Geometry check sheet. Reference: the model listing, model coordinates, mm. Face numbers are marked on the shaded views. A direction names the side the tool comes from. Give positions to 0.01 mm unless a question says otherwise; leave off trailing zeros. Write each loop counter-clockwise with the first axis right and the second up, starting at its lowest first coordinate (ties: lowest second). Pieces come first, ordered by that corner, then holes. Notation, with made-up numbers: M -37,31.25 L -23,31.25 A32 ccw -23,69.25 Z; hole C 8,82.25 d7. An arc over 180 degrees is marked long. One line per item, written item: value. Start each with the question number.
1. Tool access check on the marked faces 1, 2 and 3. Record the directions out of +Z, -Z, +X, -X, +Y, -Y that give a thin tool (end or side, any length) a straight path to the whole face; none if there is none.
2. Cross-section at C-C on z = -3. Record the cut outline in (x, y).
3. Cross-section at A-A on x = 94. Record the cut outline in (y, z) (3 decimals), then the cut area to 4 significant figures.
4. Cross-section at B-B on y = 4.5. Record the cut outline in (x, z) (3 decimals).
5. Scan lines: line 1 (Y direction, x = 6, z = 2.2) (3 decimals); line 2 (Y direction, x = 94, z = 4.2); line 3 (Z direction, x = 62.5, y = 10.75). Record each from-to range of solid material in increasing order.
6. Gauge pin test, flat ends, axial feed: pin 1 (3.5 mm diameter, centred on y = 5.5, z = -1.5, fed in from +X); pin 2 (6 mm diameter, centred on y = 2, z = -4, fed in from +X); pin 3 (5 mm diameter, centred on y = 8, z = -4.5, fed in from -X); pin 4 (4.5 mm diameter, centred on x = 91.5, y = 3, fed in from -Z). Record the tip position at first contact, or that the pin passes through.
Autodesk Inventor part; units mm, degrees
ref_plane "YZ Plane" through (0, 0, 0) normal (1, 0, 0) x (0, 1, 0)
ref_plane "XZ Plane" through (0, 0, 0) normal (0, 1, 0) x (-1, 0, 0)
ref_plane "XY Plane" through (0, 0, 0) normal (0, 0, 1) x (1, 0, 0)
sketch "Sketch1" plane through (0, 0, 0) normal (0, 0, 1) x (1, 0, 0)
  line L0 (0, 0) -> (100, 0)
  line L1 (100, 0) -> (100, 9)
  line L2 (88, 12) -> (12, 12)
  line L3 (0, 9) -> (0, 0)
  line L4 (12, 12) -> (12, 9)
  line L5 (12, 9) -> (0, 9)
  line L6 (88, 12) -> (88, 9)
  line L7 (88, 9) -> (100, 9)
  dimension "d6" = 100
  dimension "d7" = 3
  dimension "d8" = 3
  dimension "d9" = 12
  dimension "d10" = 12
  dimension "d11" = 9
  dimension "d12" = 9
  dimension "d13" = 12
extrude "Extrusion1" add sketch "Sketch1" along normal blind 6
sketch "Sketch2" plane through (0, 0, 0) normal (0, 0, -1) x (-1, 0, 0)
  line L0 (-88, 12) -> (-12, 12)
  line L1 (0, 0) -> (-100, 0)
  line L2 (-88, 12) -> (-12, 12)
  line L3 (-12, 12) -> (-12, 0)
  line L4 (-12, 0) -> (-88, 0)
  line L5 (-88, 0) -> (-88, 12)
extrude "Extrusion2" add sketch "Sketch2" along normal blind 6
sketch "Sketch3" plane through (0, 0, 0) normal (0, 0, -1) x (-1, 0, 0)
  circle A0 centre (-6, 4.5) radius 1.725
  line L0 (-12, 9) -> (0, 9)
  line L1 (0, 9) -> (0, 0)
  circle A1 centre (-94, 4.5) radius 1.725
  line L2 (-88, 0) -> (-100, 0)
  line L3 (-100, 0) -> (-100, 9)
  dimension "d18" = 3.45
  dimension "d19" = 4.5
  dimension "d20" = 6
  dimension "d21" = 3.45
  dimension "d22" = 4.5
  dimension "d23" = 6
extrude "Extrusion3" cut sketch "Sketch3" against normal blind 3
sketch "Sketch4" plane through (0, 0, 6) normal (0, 0, 1) x (1, 0, 0)
  circle A0 centre (6, 4.5) radius 3
  line L0 (12, 9) -> (0, 9)
  line L1 (0, 9) -> (0, 0)
  circle A1 centre (94, 4.5) radius 1.725
  circle A2 centre (94, 4.5) radius 3
  dimension "d26" = 6
  dimension "d27" = 4.5
  dimension "d28" = 6
  dimension "d29" = 6
extrude "Extrusion4" cut sketch "Sketch4" against normal blind 3 contours A0 | A1 | A2
fillet "Fillet1" radius 1.5 2 edges at (50, 12, 6) (50, 12, -6)
equation "\"d8\" = d7"
equation "\"d10\" = d9"
equation "\"d12\" = d11"
properties part number "beam10cm"
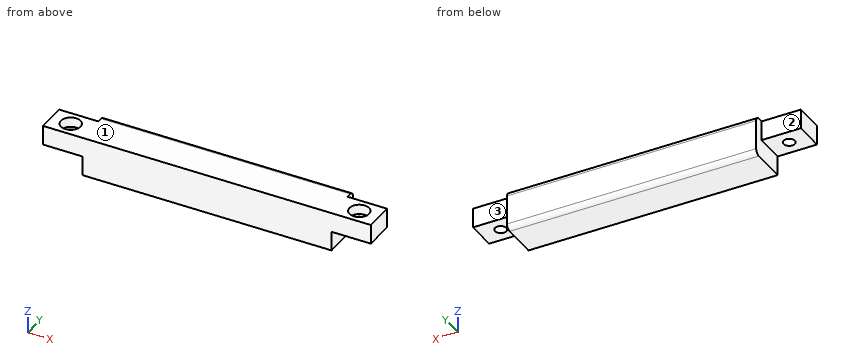
Report:
1. face 1: +Z, +X, -X, +Y, -Y
1. face 2: +Z, -Z, -X, +Y
1. face 3: +Z, -Z, +X, +Y
2. outline: M 12,0 L 88,0 L 88,12 L 12,12 Z
3. outline: M 0,0 L 2.775,0 L 2.775,3 L 1.5,3 L 1.5,6 L 0,6 Z; M 6.225,0 L 9,0 L 9,6 L 7.5,6 L 7.5,3 L 6.225,3 Z
3. area: 25.65 mm^2
4. outline: M 0,0 L 4.275,0 L 4.275,3 L 3,3 L 3,6 L 0,6 Z; M 7.725,0 L 12,0 L 12,-6 L 88,-6 L 88,0 L 92.275,0 L 92.275,3 L 91,3 L 91,6 L 9,6 L 9,3 L 7.725,3 Z; M 95.725,0 L 100,0 L 100,6 L 97,6 L 97,3 L 95.725,3 Z
5. line 1: y = 0 to 2.775, 6.225 to 9
5. line 2: y = 0 to 1.5, 7.5 to 9
5. line 3: z = -5.98 to 5.98
6. pin 1: stops at x = 100
6. pin 2: stops at x = 88
6. pin 3: stops at x = 12
6. pin 4: stops at z = 0
